Build history of the part. All positions in model axes, mm. Coordinates: 2 decimals unless noted, no trailing zeros. Write each loop counter-clockwise with the first axis right and the second up, starting at its lowest first coordinate (ties: lowest second). Pieces come first, ordered by that corner, then holes.
```python
from build123d import *

# Parameters (mm, degrees)
SCHIZZO1_R                   = 40
ESTRUSIONE_ESTRUSIONE1_DEPTH = 7
RACCORDO1_R                  = 5
SCHIZZO2_R                   = 1.5
TAGLIO_ESTRUSIONE1_DEPTH     = 37
SCHIZZO3_R                   = 1
TAGLIO_ESTRUSIONE2_DEPTH     = 10
SCHIZZO4_R                   = 1.5
TAGLIO_ESTRUSIONE3_DEPTH     = 10


with BuildPart() as part:
    # Schizzo1 → Estrusione-Estrusione1 (new body)
    with BuildSketch(Plane.XY):
        Circle(SCHIZZO1_R)
    extrude(amount=ESTRUSIONE_ESTRUSIONE1_DEPTH)

    # Raccordo1
    raccordo1_edges = [part.edges().sort_by_distance(p)[0] for p in [
        (-40, 0, 7),
    ]]
    fillet(raccordo1_edges, radius=RACCORDO1_R)

    # Schizzo2 → Taglio-Estrusione1 (cut)
    with BuildSketch(Plane.XY.offset(7)):
        with Locations((0, 25)):
            Circle(SCHIZZO2_R)
        with Locations((0, -25)):
            Circle(SCHIZZO2_R)
    extrude(amount=-TAGLIO_ESTRUSIONE1_DEPTH, mode=Mode.SUBTRACT)

    # Schizzo3 → Taglio-Estrusione2 (cut)
    with BuildSketch(Plane.XY.offset(7)):
        with Locations((0, 10.75)):
            Circle(SCHIZZO3_R)
        with Locations((0, -10.75)):
            Circle(SCHIZZO3_R)
    extrude(amount=-TAGLIO_ESTRUSIONE2_DEPTH, mode=Mode.SUBTRACT)

    # Schizzo4 → Taglio-Estrusione3 (cut)
    with BuildSketch(Plane.XY.offset(7)):
        Circle(SCHIZZO4_R)
    extrude(amount=-TAGLIO_ESTRUSIONE3_DEPTH, mode=Mode.SUBTRACT)


solid = part.part
```
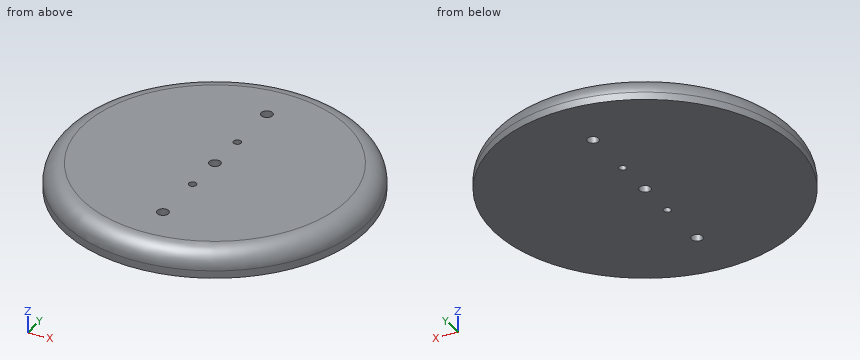
1. Probe line 1 along Y through (x, z) = (0, 2); line 2 along Y through (x, z) = (0, 3.75); line 3 along Z through (x, y) = (-35, -3). List the from-to ranges inside material, lowest first.
Computed values:
line 1: y = -40 to -26.5, -23.5 to -11.75, -9.75 to -1.5, 1.5 to 9.75, 11.75 to 23.5, 26.5 to 40
line 2: y = -39.68 to -26.5, -23.5 to -11.75, -9.75 to -1.5, 1.5 to 9.75, 11.75 to 23.5, 26.5 to 39.68
line 3: z = 0 to 7
2. Saw through at A-A on x = 0. List the corners of the cut face in (y, z), plus the area to 3 significant figures.
Computed values:
outline: (-40, 0) - (-26.5, 0) - (-26.5, 7) - (-35, 7) arc R5 ccw to (-40, 2) - close; (-23.5, 0) - (-11.75, 0) - (-11.75, 7) - (-23.5, 7) - close; (-9.75, 0) - (-1.5, 0) - (-1.5, 7) - (-9.75, 7) - close; (1.5, 0) - (9.75, 0) - (9.75, 7) - (1.5, 7) - close; (11.75, 0) - (23.5, 0) - (23.5, 7) - (11.75, 7) - close; (26.5, 0) - (40, 0) - (40, 2) arc R5 ccw to (35, 7) - (26.5, 7) - close
area: 458 mm2
3. Saw through at B-B on z = 6. List the corners of the cut face in (x, y).
Computed values:
outline: circle Ø76 at (0, 0); hole circle Ø3 at (0, -25); hole circle Ø3 at (0, 0); hole circle Ø3 at (0, 25); hole circle Ø2 at (0, -10.75); hole circle Ø2 at (0, 10.75)
4. Flat gauge pins, fed straight in: pin 1 (1.5 mm diameter, centred on x = 6.5, z = 4.5, fed in from -Y); pin 2 (1 mm diameter, centred on x = -22, z = 6, fed in from -Y); pin 3 (2 mm diameter, centred on x = -20.5, z = 1, fed in from -Y). Where does each tip first touch, or does it go through?
Computed values:
pin 1: stops at y = -39.17
pin 2: stops at y = -31.77
pin 3: stops at y = -34.92
